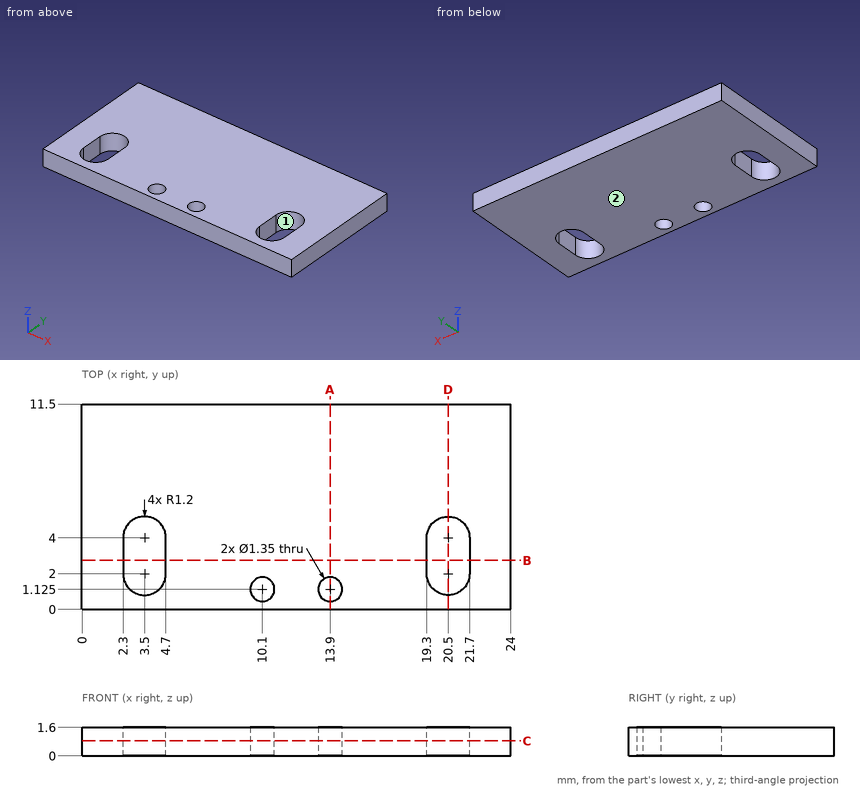
Can you work these out from the drawing? Everything is in mm from the part's minimum corner. A direction names the side the tool comes from. Round coordinates to 2 decimals unless told otherwise and drop trailing zeros. Loops run counter-clockwise (first coordinate to the right, second up) from the corner with the lowest first, then second, coordinate; pieces in that order, holes last. Notation, with made-up numbers: M 47.25,-26.5 L 69.25,-26.5 A16 cw 69.25,-4.5 Z; hole C 37,-1 d10. An arc over 180 degrees is marked long. Write item = value, one per line.
1. I want a section at A-A, the plane x = 13.9. Write out the boundary of the cut face in (y, z).
Results below:
outline = M 0,0 L 0.45,0 L 0.45,1.6 L 0,1.6 Z; M 1.8,0 L 11.5,0 L 11.5,1.6 L 1.8,1.6 Z
2. I want a section at D-D, the plane x = 20.5. Write out the boundary of the cut face in (y, z).
Results below:
outline = M 0,0 L 0.8,0 L 0.8,1.6 L 0,1.6 Z; M 5.2,0 L 11.5,0 L 11.5,1.6 L 5.2,1.6 Z
3. I want a section at B-B, the plane y = 2.75. Write out the boundary of the cut face in (x, z), and give its area (3 significant figures).
Results below:
outline = M 0,0 L 2.3,0 L 2.3,1.6 L 0,1.6 Z; M 4.7,0 L 19.3,0 L 19.3,1.6 L 4.7,1.6 Z; M 21.7,0 L 24,0 L 24,1.6 L 21.7,1.6 Z
area = 30.7 mm²
4. I need wall thicknesses on probe 1 along X at (y, z) = (3.5, 0.3); probe 2 along Y at (x, z) = (13.9, 0.4); probe 3 along X at (y, z) = (4.75, 1.2). Which ranges of each line are inside material? Lowest first, please.
Results below:
probe_1 = 0 to 2.3, 4.7 to 19.3, 21.7 to 24
probe_2 = 0 to 0.45, 1.8 to 11.5
probe_3 = 0 to 2.56, 4.44 to 19.56, 21.44 to 24
5. Which directions (+Z, -Z, +X, -X, +Y, -Y) give clear straight access to the entire face, cutting with the end or side of a thin tool? Please do the marked faces 1 and 2.
Results below:
face_1 = +Z, -Z
face_2 = -Z, +X, -X, +Y, -Y
6. I want a section at C-C, the plane z = 0.85. Write out the boundary of the cut face in (x, y) (3 decimals), and give its area (4 significant figures).
Results below:
outline = M 0,0 L 24,0 L 24,11.5 L 0,11.5 Z; hole M 2.3,2 A1.2 ccw 4.7,2 L 4.7,4 A1.2 ccw 2.3,4 Z; hole C 10.1,1.125 d1.35; hole C 13.9,1.125 d1.35; hole M 19.3,2 A1.2 ccw 21.7,2 L 21.7,4 A1.2 ccw 19.3,4 Z
area = 254.5 mm²
7. Will this pin go through, and if not, where does the flat tip stop? P1, Ø1.2, axis at x = 13.9, y = 1.125, coming from the -Z side.
Results below:
P1 = through
